from build123d import *

# Parameters (mm, degrees)
SKETCH048_W      = 3.5
SKETCH048_H      = 4
EXTRUDE045_DEPTH = 8
SKETCH044_W      = 4
SKETCH044_H      = 10
EXTRUDE041_DEPTH = 1


with BuildPart() as extrude045:
    # Sketch048 → Extrude045 (new body)
    with BuildSketch(Plane.XY):
        with Locations((0, -36)):
            Rectangle(SKETCH048_W, SKETCH048_H)
    extrude(amount=EXTRUDE045_DEPTH)


with BuildPart() as bevel004:
    # Sweep002: sweep along a path in Sketch041
    with BuildLine(Plane(origin=(0, 0, -2), x_dir=(1, 0, 0), z_dir=(0, 0, -1))) as sweep002_path:
        Line((-25, 35), (25, 35))
        ThreePointArc((25, 35), (27.12132, 34.12132), (28, 32))
        Line((28, 32), (28, -32))
        ThreePointArc((28, -32), (27.12132, -34.12132), (25, -35))
        Line((25, -35), (-25, -35))
        ThreePointArc((-25, -35), (-27.12132, -34.12132), (-28, -32))
        Line((-28, -32), (-28, 32))
        ThreePointArc((-28, 32), (-27.12132, 34.12132), (-25, 35))
    # Sketch040 → Sweep002 (sweep)
    with BuildSketch(Plane.XZ):
        Polygon((-28, 11), (-30, 9), (-30, 1), (-28, -1), (-28, -2), (-33, -2), (-33, 12), (-28, 12), align=None)
    sweep(path=sweep002_path.line)


with BuildPart() as compound:
    # Sketch044 → Extrude041 (new body)
    with BuildSketch(Plane.XY.offset(7)):
        with Locations((-29, 21)):
            Rectangle(SKETCH044_W, SKETCH044_H)
    extrude(amount=EXTRUDE041_DEPTH)

    # Compound: union bevel004
    add(bevel004.part)


with BuildPart() as cut039:
    # Sweep001: sweep along a path in Sketch038
    with BuildLine(Plane(origin=(0, 0, 0), x_dir=(1, 0, 0), z_dir=(0, 0, -1))) as sweep001_path:
        Line((-25, 35), (25, 35))
        ThreePointArc((25, 35), (27.12132, 34.12132), (28, 32))
        Line((28, 32), (28, -32))
        ThreePointArc((28, -32), (27.12132, -34.12132), (25, -35))
        Line((25, -35), (-25, -35))
        ThreePointArc((-25, -35), (-27.12132, -34.12132), (-28, -32))
        Line((-28, -32), (-28, 32))
        ThreePointArc((-28, 32), (-27.12132, 34.12132), (-25, 35))
    # Sketch037 → Sweep001 (sweep)
    with BuildSketch(Plane(origin=(0, 0, 0), x_dir=(-1, 0, 0), z_dir=(0, 1, 0))):
        Polygon((-30, 8), (-29.1, 8), (-29.1, 6), (-28, 6), (-28, 0), (-30, 0), align=None)
    sweep(path=sweep001_path.line)

    # Cut037: cut Compound
    add(compound.part, mode=Mode.SUBTRACT)

    # Cut039: cut Extrude045
    add(extrude045.part, mode=Mode.SUBTRACT)


solid = cut039.part
Geometry: final body of the model. Coordinates: model frame, mm. A direction names the side the tool comes from. Give positions to 0.01 mm unless a question says otherwise; leave off trailing zeros. Write each loop counter-clockwise with the first axis right and the second up, starting at its lowest first coordinate (ties: lowest second). Pieces come first, ordered by that corner, then holes. Notation, with made-up numbers: (46, 50) -> (70, 50) arc R21 ccw to (70, 56) -> close; hole circle Ø3 at (-24, 26.5). An arc over 180 degrees is marked (long way). Answer as a JSON object with one key per item and string values.
1. Ray query, probe 1 along X at (y, z) = (26, 4); probe 2 along X at (y, z) = (7, 7.5); probe 3 along Y at (x, z) = (-7, 1). Return the intervals inside material, ascending. Write a range as from..to.
Ans:
{"probe 1": "x = -30..-28, 28..30", "probe 2": "x = -30..-29.1, 29.1..30", "probe 3": "y = -37..-35, 35..37"}
2. Cut plane B-B on x = 13.5. Output: boundary loops of the cut face in (y, z), and give its area (3 significant figures).
Ans:
{"outline": "(-37, 1) -> (-36, 0) -> (-35, 0) -> (-35, 6) -> (-36.1, 6) -> (-36.1, 8) -> (-37, 8) -> close; (35, 0) -> (36, 0) -> (37, 1) -> (37, 8) -> (36.1, 8) -> (36.1, 6) -> (35, 6) -> close", "area": "26.6 mm^2"}
3. Cut plane A-A on y = 20.5. Output: boundary loops of the cut face in (x, z).
Ans:
{"outline": "(-30, 1) -> (-29, 0) -> (-28, 0) -> (-28, 6) -> (-29.1, 6) -> (-29.1, 7) -> (-30, 7) -> close; (28, 0) -> (29, 0) -> (30, 1) -> (30, 8) -> (29.1, 8) -> (29.1, 6) -> (28, 6) -> close"}
4. Access query for faces 1 (the flat face through (14, -35, 3)), 2 (the cylindrical face through (28, -36, 4)), 3 (the flat face through (29.1, 0, 7)), 4 (the flat face through (1.75, -36, 4)), 5 (the flat face through (14, -37, 5)). Directions: +Z, -Z, +X, -X, +Y, -Y. A direction counts if a zero-diameter tool reaches every point of the face in a straight line with its end or side. Return the directions, or none.
Ans:
{"face 1": "+Z, -Z", "face 2": "+Z, -Z, +X, -Y", "face 3": "+Z", "face 4": "+Z, -Z, -Y", "face 5": "+Z, -Z, +X, -X, -Y"}
5. Mould query, pull axis X, two halves, no side actions, for faces 6 (the cylindrical face through (27.9, -34.9, 7)), 7 (the conical face through (28.063, 34.996, 0.285)), 8 (the flat face through (-29.4, -10.4, 8)). Classes: pulls with the +X half, pulls with the -X half, needs draft (parallel to the pull), parting line crosses it, or undercut.
Ans:
{"face 6": "undercut", "face 7": "pulls with the +X half", "face 8": "needs draft"}
6. Contact query for flat-ended pins moving along their axis: pin 1 (1 mm diameter, centred on x = -29.5, z = 7.5, fed in from -Y); pin 2 (2 mm diameter, centred on y = -36, z = 4, fed in from -X); pin 3 (0.7 mm diameter, centred on x = -29.5, y = 19.5, fed in from +Z). Output: stop coordinate, or through.
Ans:
{"pin 1": "stops at y = -35", "pin 2": "stops at x = -29", "pin 3": "stops at z = 7"}
